Here's the drawing with two shaded views (mm, measured from the low corner). I have some questions. A direction names the side the tool comes from. Coordinates: 2 decimals unless noted, no trailing zeros. Order: outer loops, then holes, each group sorted by start corner. A loop starts at its lowest first (then second) coordinate and runs counter-clockwise, first axis right, second up. Notation, with made-up numbers: (26.25, 28.5) -> (38.25, 28.5) arc R11 cw to (38.25, 32.5) -> close; hole circle Ø5 at (-36.75, 76.25). An arc over 180 degrees is marked (long way). Write item = value, one per line.
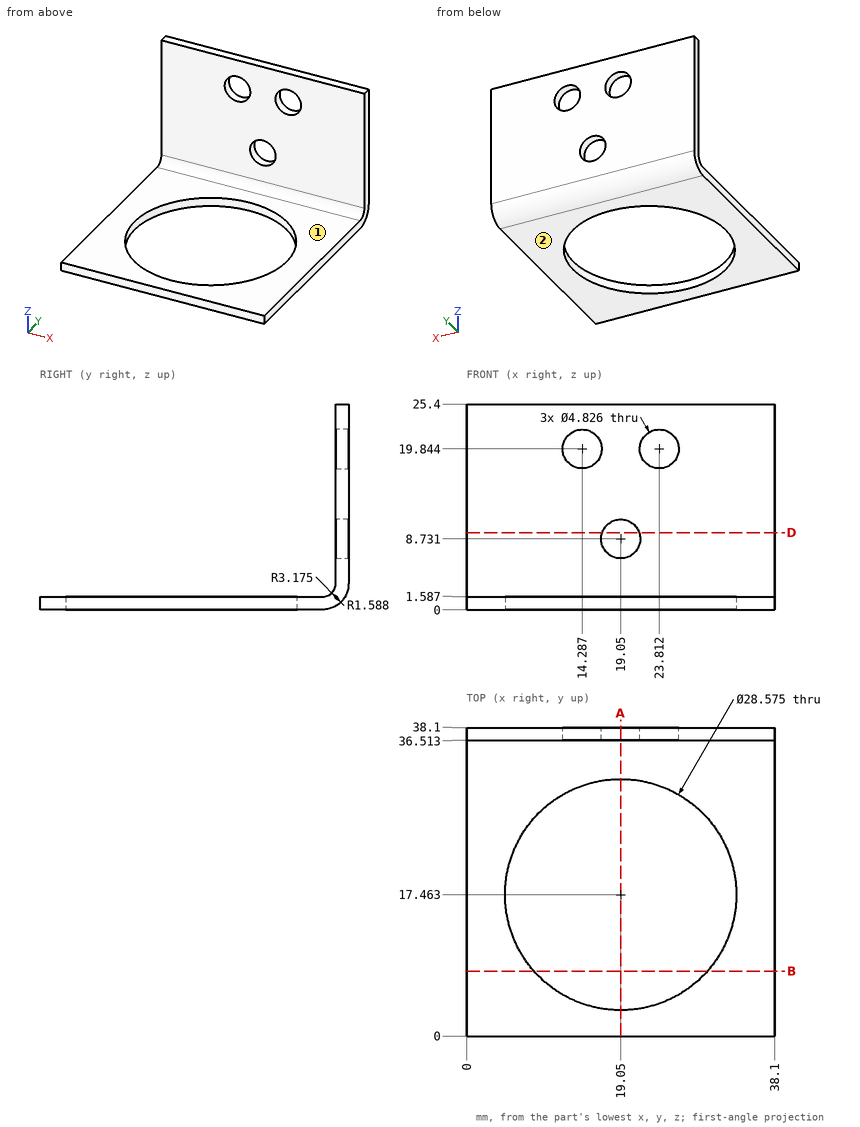
Item 1: If I drill on probe 1 along Z at (x, y) = (28.5, 35); probe 2 along Y at (x, z) = (23.5, 3.5); probe 3 along Z at (x, y) = (19, 37) (1 decimal), over which ranges is the centre line in solid material (lowest first)?
A:
probe_1 = 0 to 1.59
probe_2 = 36.51 to 38.1
probe_3 = 0.8 to 6.3, 11.1 to 25.4
Item 2: For the marked faces 1 and 2, which set-ups out of +Z, -Z, +X, -X, +Y, -Y let a thin tool reach every point of the face, with its end or its side?
A:
face_1 = +Z, +X, -X, -Y
face_2 = -Z, +X, -X, +Y, -Y
Item 3: I'm going to push flat-ended pins straight in: P1, Ø17.5, axis at x = 18, y = 10, coming from the +Z side; P2, Ø7.5, axis at x = 19.05, z = 8.73, coming from the -Y side; P3, Ø4, axis at x = 14.29, z = 19.84, coming from the -Y side; P4, Ø10, axis at x = 12.5, z = 20, coming from the +Y side. Where does each tip first touch, or does it pass through?
A:
P1 = 1.59
P2 = 36.51
P3 = through
P4 = 38.1
Item 4: I want a section at B-B, the plane y = 8. Please give me the cut outline in (x, z) (1 decimal), plus the area to 3 significant figures.
A:
outline = (0, 0) -> (8.3, 0) -> (8.3, 1.6) -> (0, 1.6) -> close; (29.8, 0) -> (38.1, 0) -> (38.1, 1.6) -> (29.8, 1.6) -> close
area = 26.5 mm2
Item 5: I want a section at D-D, the plane z = 9.5. Please give me the cut outline in (x, y).
A:
outline = (0, 36.51) -> (16.76, 36.51) -> (16.76, 38.1) -> (0, 38.1) -> close; (21.34, 36.51) -> (38.1, 36.51) -> (38.1, 38.1) -> (21.34, 38.1) -> close
Item 6: I want a section at A-A, the plane x = 19.05. Give the number of separate pieces and of enclosed holes in the cut face.
A:
separate_pieces = 3
enclosed_holes = 0
